Check sheet for the modelled part. Datum: model origin and axes. Units: mm. Face numbers are marked on the shaded views. A direction names the side the tool comes from. Give positions to 0.01 mm unless a question says otherwise; leave off trailing zeros. Write each loop counter-clockwise with the first axis right and the second up, starting at its lowest first coordinate (ties: lowest second). Pieces come first, ordered by that corner, then holes. Notation, with made-up numbers: (67, 51.25) - (76, 51.25) arc R17 cw to (76, 77.25) - close; hole circle Ø6 at (-15, -18). An arc over 180 degrees is marked (long way). Return JSON: item names as keys, results as strings. Group by question number.
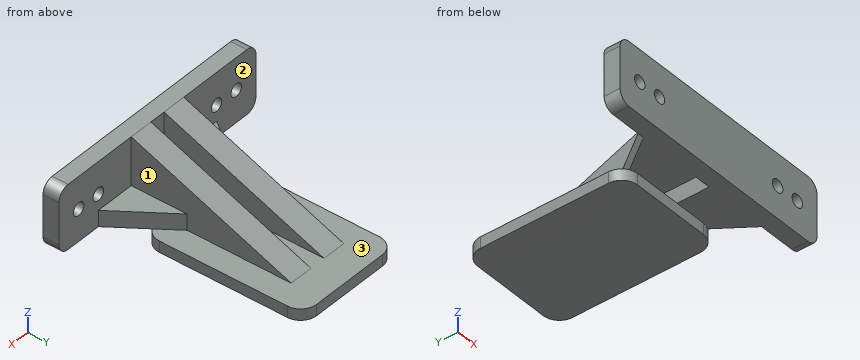
Autodesk Inventor part; units mm, degrees
ref_plane "Work Plane1" through (-20, -40, 0) normal (-1, 0, 0) x (0, 0, 1)
ref_plane "YZ Plane" through (0, 0, 0) normal (1, 0, 0) x (0, 1, 0)
ref_plane "XZ Plane" through (0, 0, 0) normal (0, 1, 0) x (-1, 0, 0)
sketch "Sketch1" plane through (0, 0, 0) normal (0, 0, 1) x (1, 0, 0)
  line L0 (35, -50) -> (-35, -50)
  line L1 (-35, -50) -> (-35, 50)
  line L2 (-35, 50) -> (35, 50)
  line L3 (35, 50) -> (35, -50)
  line L4 (35, -50) -> (-35, 50) construction
  line L5 (-35, -50) -> (35, 50) construction
  point P0 (0, 0)
  dimension "d0" = 70
  dimension "d1" = 100
extrude "Extrusion1" add sketch "Sketch1" along normal blind 7
fillet "Fillet1" radius 10 4 edges at (35, 50, 3.5) (-35, 50, 3.5) (-35, -50, 3.5) (35, -50, 3.5)
ref_plane "Work Plane1" through (-20, -40, 0) normal (-1, 0, 0) x (0, 0, 1)
sketch "Sketch2" plane through (-20, -40, 0) normal (-1, 0, 0) x (0, 0, 1)
  line L0 (7, 80) -> (7, 90) construction
  line L1 (7, 90) -> (0, 90) construction
  line L2 (0, 90) -> (0, 80) construction
  line L3 (0, 80) -> (7, 80) construction
  line L4 (7, 0) -> (0, 0) construction
  line L5 (7, 80) -> (7, 0) construction
  line L6 (0, 80) -> (7, 80) construction
  line L7 (0, 0) -> (0, 80) construction
  line L8 (7, -10) -> (7, 0) construction
  line L9 (7, 0) -> (0, 0) construction
  line L10 (0, 0) -> (0, -10) construction
  line L11 (0, -10) -> (7, -10) construction
  line L12 (0, -10) -> (7, -10) construction
  line L13 (57, 70) -> (7, 70) construction
  line L14 (7, 70) -> (7, -10) construction
  line L15 (7, 70) -> (47, 70) construction
  line L16 (47, 70) -> (47, -30) construction
  line L17 (47, -30) -> (7, -30) construction
  line L18 (7, -30) -> (7, 70) construction
  line L19 (7, 70) -> (7, -30)
  line L20 (7, -30) -> (47, -30)
  line L21 (47, -30) -> (7, 70)
  line L22 (0, 0) -> (7, 0) construction
  line L23 (0, 80) -> (0, 0) construction
  line L24 (7, 80) -> (0, 80) construction
  line L25 (7, 0) -> (7, 80) construction
  line L26 (7, 90) -> (7, 80) construction
  line L27 (7, 80) -> (0, 80) construction
  line L28 (0, 80) -> (0, 90) construction
  line L29 (0, 90) -> (7, 90) construction
  line L30 (7, 0) -> (7, -10) construction
  line L31 (7, -10) -> (0, -10) construction
  line L32 (0, -10) -> (0, 0) construction
  line L33 (0, 0) -> (7, 0) construction
  point P0 (0, 40)
  dimension "d6" = 50
  dimension "d8" = 40
  dimension "d9" = 100
  dimension "d17" = 20
extrude "Extrusion2" add sketch "Sketch2" against normal blind 40
sketch "Sketch3" plane through (-20, -70, 7) normal (0, -1, 0) x (1, 0, 0)
  line L0 (0, 0) -> (0, 40) construction
  line L1 (0, 0) -> (40, 0) construction
  line L2 (40, 40) -> (40, 0) construction
  line L3 (0, 40) -> (40, 40) construction
  line L4 (0, 40) -> (-55, 40) construction
  line L5 (-55, 40) -> (95, 40)
  line L6 (95, 40) -> (95, 0)
  line L7 (95, 0) -> (-55, 0)
  line L8 (-55, 0) -> (-55, 40)
  point P0 (20, -7)
  dimension "d12" = 55
  dimension "d13" = 150
  dimension "d18" = 40
extrude "Extrusion3" add sketch "Sketch3" along normal blind 10
fillet "Fillet2" radius 7 4 edges at (-75, -75, 47) (75, -75, 47) (75, -75, 7) (-75, -75, 7)
sketch "Sketch5" plane through (-20, -80, 7) normal (0, -1, 0) x (1, 0, 0)
  arc A0 (-55, 7) -> (-48, 0) centre (-48, 7) ccw construction
  line L0 (-48, 0) -> (88, 0) construction
  arc A1 (88, 0) -> (95, 7) centre (88, 7) ccw construction
  line L1 (95, 7) -> (95, 33) construction
  arc A2 (95, 33) -> (88, 40) centre (88, 33) ccw construction
  line L2 (88, 40) -> (-48, 40) construction
  arc A3 (-48, 40) -> (-55, 33) centre (-48, 33) ccw construction
  line L3 (-55, 33) -> (-55, 7) construction
  line L4 (95, 20) -> (-55, 20) construction
  line L5 (-55, 7) -> (-55, 33) construction
  line L6 (0, 0) -> (40, 0) construction
  line L7 (20, 0) -> (20, 40) construction
  circle A4 centre (80, 20) radius 4
  circle A5 centre (-40, 20) radius 4
  circle A6 centre (65, 20) radius 4
  circle A7 centre (-25, 20) radius 4
  point P0 (20, -7)
  dimension "d23" = 8
  dimension "d24" = 8
  dimension "d25" = 15
  dimension "d26" = 15
  dimension "d29" = 8
  dimension "d30" = 8
  dimension "d31" = 15
  dimension "d32" = 15
extrude "Extrusion4" cut sketch "Sketch5" against normal blind 20
sketch "Sketch7" plane through (-20, -70, 47) normal (0, 0, 1) x (1, 0, 0)
  line L0 (0, 0) -> (0, 100) construction
  line L1 (0, 0) -> (40, 0) construction
  line L2 (40, 100) -> (40, 0) construction
  line L3 (0, 100) -> (40, 100) construction
  line L4 (20, 100) -> (20, 0) construction
  line L5 (0, 20) -> (0, 100) construction
  line L6 (0, 50) -> (20, 50) construction
  line L7 (25, 0) -> (15, 0)
  line L8 (15, 0) -> (15, 100)
  line L9 (15, 100) -> (25, 100)
  line L10 (25, 100) -> (25, 0)
  line L11 (25, 0) -> (15, 100) construction
  line L12 (15, 0) -> (25, 100) construction
  point P0 (20, 70)
  dimension "d33" = 10
extrude "Extrusion5" cut sketch "Sketch7" against normal blind 40
sketch "Sketch8" plane through (0, 0, 7) normal (0, 0, 1) x (1, 0, 0)
  line L0 (-20, -50) -> (-20, 30) construction
  line L1 (-20, 30) -> (-5, 30) construction
  line L2 (-5, -50) -> (-5, 30) construction
  line L3 (-5, -50) -> (5, -50) construction
  line L4 (5, 30) -> (5, -50) construction
  line L5 (5, 30) -> (20, 30) construction
  line L6 (20, 30) -> (20, -50) construction
  line L7 (20, -50) -> (25, -50) construction
  arc A0 (25, -50) -> (35, -40) centre (25, -40) ccw construction
  line L8 (35, -40) -> (35, 40) construction
  arc A1 (35, 40) -> (25, 50) centre (25, 40) ccw construction
  line L9 (25, 50) -> (-25, 50) construction
  arc A2 (-25, 50) -> (-35, 40) centre (-25, 40) ccw construction
  line L10 (-35, 40) -> (-35, -40) construction
  arc A3 (-35, -40) -> (-25, -50) centre (-25, -40) ccw construction
  line L11 (-25, -50) -> (-20, -50) construction
  line L12 (-5, -70) -> (-5, 30) construction
  line L13 (-20, 30) -> (-5, 30) construction
  line L14 (-20, -70) -> (-20, 30) construction
  line L15 (-20, -70) -> (-5, -70) construction
  line L16 (5, 30) -> (5, -70) construction
  line L17 (5, -70) -> (20, -70) construction
  line L18 (20, 30) -> (20, -70) construction
  line L19 (5, 30) -> (20, 30) construction
  line L20 (68, -70) -> (68, -80) construction
  line L21 (20, -70) -> (68, -70) construction
  line L22 (5, -70) -> (20, -70) construction
  line L23 (-5, -70) -> (5, -70) construction
  line L24 (-20, -70) -> (-5, -70) construction
  line L25 (-68, -70) -> (-20, -70) construction
  line L26 (-68, -80) -> (-68, -70) construction
  line L27 (68, -80) -> (-68, -80) construction
  line L28 (-20, -70) -> (-45, -70)
  line L29 (-20, -70) -> (-20, -35)
  line L30 (-20, -35) -> (-45, -70)
  line L31 (25, -50) -> (-25, -50) construction
  line L32 (0, -50) -> (0, -70) construction
  line L33 (20, -70) -> (45, -70)
  line L34 (20, -70) -> (20, -35)
  line L35 (20, -35) -> (45, -70)
  point P0 (0, 0)
  dimension "d0" = 70
  dimension "d36" = 25
  dimension "d37" = 35
extrude "Extrusion6" add sketch "Sketch8" along normal blind 10
properties part number "Mordaza"
Item 1: Section check B-B on z = 27. Record the cut outline in (x, y).
Item 2: Section check A-A on x = -60. Record the cut outline in (y, z).
Item 3: Section check D-D on z = 35. Record the cut outline in (x, y), plus the area to 3 significant figures.
Item 4: Material ranges on line 1 along Z through (x, y) = (-45, -73.75); line 2 along X through (y, z) = (-54, 25); line 3 along X through (y, z) = (9, 4), recorded low to high. Write a range as from..to.
Item 5: Depth check by flat-ended pin: pin 1 (25 mm diameter, centred on x = -18, y = -69, fed in from -Z); pin 2 (8 mm diameter, centred on y = 2, z = 16, fed in from -X); pin 3 (12 mm diameter, centred on y = -25.5, z = 19.5, fed in from +X). Enter the tip coordinate at first touch or a pass-through.
Item 6: Section check C-C on y = -4. Record the cut outline in (x, z).
Item 7: Access from +Z, -Z, +X, -X, +Y, -Y to the whole of each face (thin tool, end or side, straight path). Record for the marked faces 1, 2 and 3.
Reply:
{
 "1": {"outline": "(-75, -80) - (-64, -80) - (-64, -70) - (-75, -70) - close; (-56, -80) - (-49, -80) - (-49, -70) - (-56, -70) - close; (-41, -80) - (41, -80) - (41, -70) - (20, -70) - (20, -20) - (5, -20) - (5, -70) - (-5, -70) - (-5, -20) - (-20, -20) - (-20, -70) - (-41, -70) - close; (49, -80) - (56, -80) - (56, -70) - (49, -70) - close; (64, -80) - (75, -80) - (75, -70) - (64, -70) - close"},
 "2": {"outline": "(-80, 7) - (-70, 7) - (-70, 23) - (-80, 23) - close; (-80, 31) - (-70, 31) - (-70, 47) - (-80, 47) - close"},
 "3": {"outline": "(-75, -80) - (75, -80) - (75, -70) - (20, -70) - (20, -40) - (5, -40) - (5, -70) - (-5, -70) - (-5, -40) - (-20, -40) - (-20, -70) - (-75, -70) - close", "area": "2,400 mm²"},
 "4": {"line 1": "7..23, 31..47", "line 2": "-20..-5, 5..20", "line 3": "-35..35"},
 "5": {"pin 1": "z = 7", "pin 2": "x = -20", "pin 3": "x = 20"},
 "6": {"outline": "(-35, 0) - (35, 0) - (35, 7) - (20, 7) - (20, 20.6) - (5, 20.6) - (5, 7) - (-5, 7) - (-5, 20.6) - (-20, 20.6) - (-20, 7) - (-35, 7) - close"},
 "7": {"face 1": "+Z, +X, +Y", "face 2": "+Z, -X, +Y", "face 3": "+Z, +Y"}
}
